```python
from build123d import *

# Parameters (mm, degrees)
F0_W     = 203.2
F0_H     = 101.6
F1_DEPTH = 107.95
F2_T     = -3.175
F3_W     = 82.55
F3_H     = 25.4
F4_DEPTH = 25.4
F6_R     = 3.175
F7_DEPTH = 25.4
F8_R     = 3.175
F9_DEPTH = 25.4


with BuildPart() as f1:
    # F0 (on Top) → F1 (new body)
    with BuildSketch(Plane.XY):
        with Locations((52.650332, 50.8)):
            Rectangle(F0_W, F0_H)
    extrude(amount=F1_DEPTH)

    # F2
    f2_openings = [f1.faces().sort_by_distance(p)[0] for p in [
        (52.650332, 50.8, 107.95),
    ]]
    offset(amount=F2_T, openings=f2_openings)

    # F3 (on Front) → F4 (cut)
    with BuildSketch(Plane.XZ):
        with Locations((11.375332, 53.975)):
            Rectangle(F3_W, F3_H)
    extrude(amount=-F4_DEPTH, mode=Mode.SUBTRACT)

    # F6 (on Front) → F7 (cut)
    with BuildSketch(Plane.XZ):
        with Locations((-39.424668, 53.975)):
            Circle(F6_R)
    extrude(amount=-F7_DEPTH, mode=Mode.SUBTRACT)

    # F8 (on Front) → F9 (cut)
    with BuildSketch(Plane.XZ):
        with Locations((62.175332, 53.975)):
            Circle(F8_R)
    extrude(amount=-F9_DEPTH, mode=Mode.SUBTRACT)


solid = f1.part
```
The model under review builds one solid part; all positions refer to its coordinate system, in mm. A direction names the side the tool comes from. Give positions to 0.01 mm unless a question says otherwise; leave off trailing zeros. Write each loop counter-clockwise with the first axis right and the second up, starting at its lowest first coordinate (ties: lowest second). Pieces come first, ordered by that corner, then holes. Notation, with made-up numbers: (-22, 57) -> (32, 57) arc R13 cw to (32, 70) -> close; hole circle Ø3 at (56.25, 18). An arc over 180 degrees is marked (long way). Answer in a Markdown table with one row per item.
1) Clearance check with flat-ended pins moving along their axes: P1, Ø4, axis at x = -39.42, z = 53.98, coming from the -Y side (3 decimals); P2, Ø2, axis at x = 112, y = 60, coming from the +Z side (3 decimals). State where each tip first meets the part, or that it passes through.
Worked answers:
| item | result |
|---|---|
| P1 | y = 98.425 |
| P2 | z = 3.175 |
2) Mouldability with a two-part tool opening along Y and no side actions: class faces 4 (the flat face through (51, 0, 41)), 5 (the flat face through (51, 98.425, 55)), 6 (the flat face through (-48.95, 50, 53)) as +Y half, -Y half, draft (parallel to the pull), parting line (faces both ways), or undercut.
Worked answers:
| item | result |
|---|---|
| face 4 | -Y half |
| face 5 | undercut |
| face 6 | draft |
3) For L1, parallel to X at y = 87, z = 73.5; L2, parallel to Y at x = 37, z = 99 (3 decimals); L3, parallel to Z at x = 31, y = 72.5 (3 decimals), list the stretches that pass through material, from the lowest coordinate up. Write a range as [from, to].
Worked answers:
| item | result |
|---|---|
| L1 | [-48.95, -45.77], [151.08, 154.25] |
| L2 | [0, 3.175], [98.425, 101.6] |
| L3 | [0, 3.175] |
4) Tool access review of faces 1 (the flat face through (51, 101.6, 53)), 2 (the cylindrical face through (-41.94, 1.57, 52.04)), 3 (the flat face through (73, 3.175, 55)): name each direction out of +Z, -Z, +X, -X, +Y, -Y from which nothing blocks a thin tool from reaching the whole face with its end or side.
Worked answers:
| item | result |
|---|---|
| face 1 | +Z, -Z, +X, -X, +Y |
| face 2 | -Y |
| face 3 | +Z |
5) Add section A-A on x = 5. State the section outline as (y, z) points (3 decimals), plus the area to 3 significant figures.
Worked answers:
| item | result |
|---|---|
| outline | (0, 0) -> (101.6, 0) -> (101.6, 107.95) -> (98.425, 107.95) -> (98.425, 3.175) -> (3.175, 3.175) -> (3.175, 41.275) -> (0, 41.275) -> close; (0, 66.675) -> (3.175, 66.675) -> (3.175, 107.95) -> (0, 107.95) -> close |
| area | 907 mm² |
6) Add section D-D on y = 63. State the section outline as (x, z) points (3 decimals), plus the area to 3 significant figures.
Worked answers:
| item | result |
|---|---|
| outline | (-48.95, 0) -> (154.25, 0) -> (154.25, 107.95) -> (151.075, 107.95) -> (151.075, 3.175) -> (-45.775, 3.175) -> (-45.775, 107.95) -> (-48.95, 107.95) -> close |
| area | 1,310 mm² |
7) Add section B-B on z = 12.5. State the section outline as (x, y) points (3 decimals), plus the area to 3 significant figures.
Worked answers:
| item | result |
|---|---|
| outline | (-48.95, 0) -> (154.25, 0) -> (154.25, 101.6) -> (-48.95, 101.6) -> close; hole (-45.775, 3.175) -> (151.075, 3.175) -> (151.075, 98.425) -> (-45.775, 98.425) -> close |
| area | 1,900 mm² |
8) Add section C-C on x = 138. State the section outline as (y, z) points (3 decimals), plus the area to 3 significant figures.
Worked answers:
| item | result |
|---|---|
| outline | (0, 0) -> (101.6, 0) -> (101.6, 107.95) -> (98.425, 107.95) -> (98.425, 3.175) -> (3.175, 3.175) -> (3.175, 107.95) -> (0, 107.95) -> close |
| area | 988 mm² |
